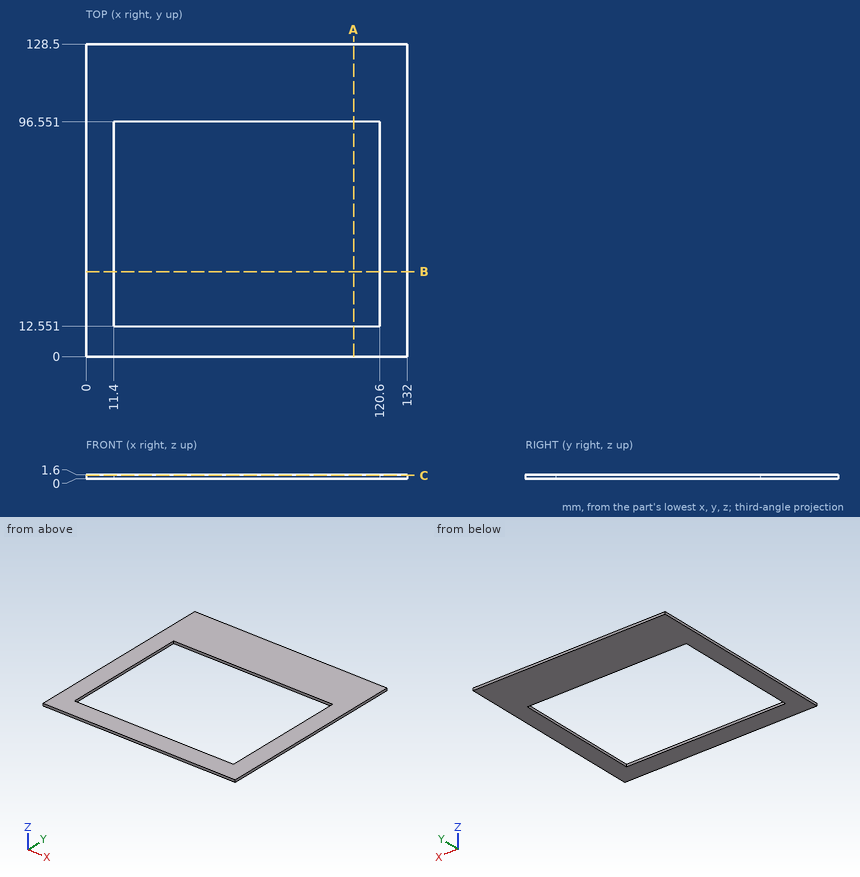
Check sheet for the drawn part. Datum: minimum x, y, z corner. Units: mm. Round coordinates to 2 decimals unless told otherwise and drop trailing zeros. Order: outer loops, then holes, each group sorted by start corner. A loop starts at its lowest first (then second) coordinate and runs counter-clockwise, first axis right, second up. Notation, with made-up numbers: (45, 59.5) -> (87, 59.5) arc R31 cw to (87, 84.5) -> close; hole circle Ø3 at (5.25, 45.5). An arc over 180 degrees is marked (long way). Put each result on its own line as item: value. Start each with the question number.
(1) Section check A-A (x = 110). Enter the section's corners in (y, z), then the cut area to 3 significant figures.
(2) Depth check by flat-ended pin: pin 1 Ø5 at (x, y) = (98, 103) entering from -Z. Enter the tip coordinate at first touch or a pass-through.
(3) Section check C-C (z = 1.3). Enter the section's corners in (x, y).
(4) Material ranges on line 1 along X through (y, z) = (17.5, 0.2); line 2 along Y through (x, z) = (55, 0.9), recorded low to high.
(5) Section check B-B (y = 35). Enter the section's corners in (x, z).
Completed:
1. outline: (0, 0) -> (12.55, 0) -> (12.55, 1.6) -> (0, 1.6) -> close; (96.55, 0) -> (128.5, 0) -> (128.5, 1.6) -> (96.55, 1.6) -> close
1. area: 71.2 mm2
2. pin 1: stops at z = 0
3. outline: (0, 0) -> (132, 0) -> (132, 128.5) -> (0, 128.5) -> close; hole (11.4, 12.55) -> (120.6, 12.55) -> (120.6, 96.55) -> (11.4, 96.55) -> close
4. line 1: x = 0 to 11.4, 120.6 to 132
4. line 2: y = 0 to 12.55, 96.55 to 128.5
5. outline: (0, 0) -> (11.4, 0) -> (11.4, 1.6) -> (0, 1.6) -> close; (120.6, 0) -> (132, 0) -> (132, 1.6) -> (120.6, 1.6) -> close
